from build123d import *

# Parameters (mm, degrees)
F1_R     = 6.25
F2_DEPTH = 14
F0_W     = 50
F0_H     = 50
F3_DEPTH = 3
F5_D     = 6
F5_DEPTH = 12
F5_TIP   = 1.8025818571
F6_SIZE  = 1


with BuildPart() as f2:
    # F1 (on face) → F2 (new body)
    with BuildSketch(Plane.XZ):
        with Locations((25, 26.5)):
            Circle(F1_R)
    extrude(amount=F2_DEPTH)

    # F0 (on Front) → F3 (join)
    with BuildSketch(Plane.XZ):
        with Locations((25, 25)):
            Rectangle(F0_W, F0_H)
    extrude(amount=-F3_DEPTH)

    # F5
    with Locations(Plane.XZ.offset(14)):
        with Locations((25, 26.5)):
            Hole(F5_D / 2, depth=F5_DEPTH)
            with Locations((0, 0, -(F5_DEPTH + F5_TIP / 2))):  # 118° drill point
                Cone(0, F5_D / 2, F5_TIP, mode=Mode.SUBTRACT)

    # F6
    f6_edges = [f2.edges().sort_by_distance(p)[0] for p in [
        (25, 3, 50),
        (50, 3, 25),
        (0, 3, 25),
        (25, 3, 0),
    ]]
    chamfer(f6_edges, length=F6_SIZE)


solid = f2.part
The model under review builds one solid part; all positions refer to its coordinate system, in mm. A direction names the side the tool comes from. Coordinates: 2 decimals unless noted, no trailing zeros. Loops run counter-clockwise (first coordinate to the right, second up) from the corner with the lowest first, then second, coordinate; pieces in that order, holes last.
(1) Consider section A-A, the plane z = 18.5. Give the boundary of the cut face in (x, y), plus the area to 3 significant figures.
Determined:
outline: (0, 0) - (50, 0) - (50, 2) - (49, 3) - (1, 3) - (0, 2) - close
area: 149 mm2
(2) Consider section B-B, the plane y = -5. Give the boundary of the cut face in (x, z).
Determined:
outline: circle Ø12.5 at (25, 26.5); hole circle Ø6 at (25, 26.5)
(3) Insertion check: P1, Ø4, axis at x = 5.5, y = -2.5, coming from the +Z side; P2, Ø3, axis at x = 22, y = -11, coming from the -Z side; P3, Ø15, axis at x = 34.5, z = 16.5, coming from the -Y side. Each pin has a flat end and moves straight along its axis. Give the tip position at first contact, or say it passes through.
Determined:
P1: passes through
P2: stops at z = 20.43
P3: stops at y = 0
(4) Draft analysis for pull direction X (two halves, no side actions). For faces 3 (the cylindrical face through (20.39, -6.9, 30.72)), 4 (the flat face through (25, 1, 0)), 5 (the conical face through (24.5, -0.5, 26.5)), state which applies: +X half, -X half, draft (parallel to the pull), parting line (faces both ways), or undercut.
Determined:
face 3: parting line
face 4: draft
face 5: undercut
(5) Tool access review of faces 1 (the cylindrical face through (28, -7.9, 26.6)), 2 (the flat face through (25, 3, 25)): name each direction out of +Z, -Z, +X, -X, +Y, -Y from which nothing blocks a thin tool from reaching the whole face with its end or side.
Determined:
face 1: -Y
face 2: +Z, -Z, +X, -X, +Y
(6) Consider section D-D, the plane z = 31. Give the boundary of the cut face in (x, y).
Determined:
outline: (0, 0) - (20.66, 0) - (20.66, -14) - (29.34, -14) - (29.34, 0) - (50, 0) - (50, 2) - (49, 3) - (1, 3) - (0, 2) - close
(7) Wall thickness on L1, parallel to Z at x = 25, y = -10; L2, parallel to Y at x = 35.5, z = 26.5; L3, parallel to Z at x = 29, y = -4.5: over which ranges is each line inside the solid? List them lowest first.
Determined:
L1: z = 20.25 to 23.5, 29.5 to 32.75
L2: y = 0 to 3
L3: z = 21.7 to 31.3
(8) Consider section C-C, the plane x = 16. Give the boundary of the cut face in (y, z), plus the area to 3 significant figures.
Determined:
outline: (0, 0) - (2, 0) - (3, 1) - (3, 49) - (2, 50) - (0, 50) - close
area: 149 mm2
